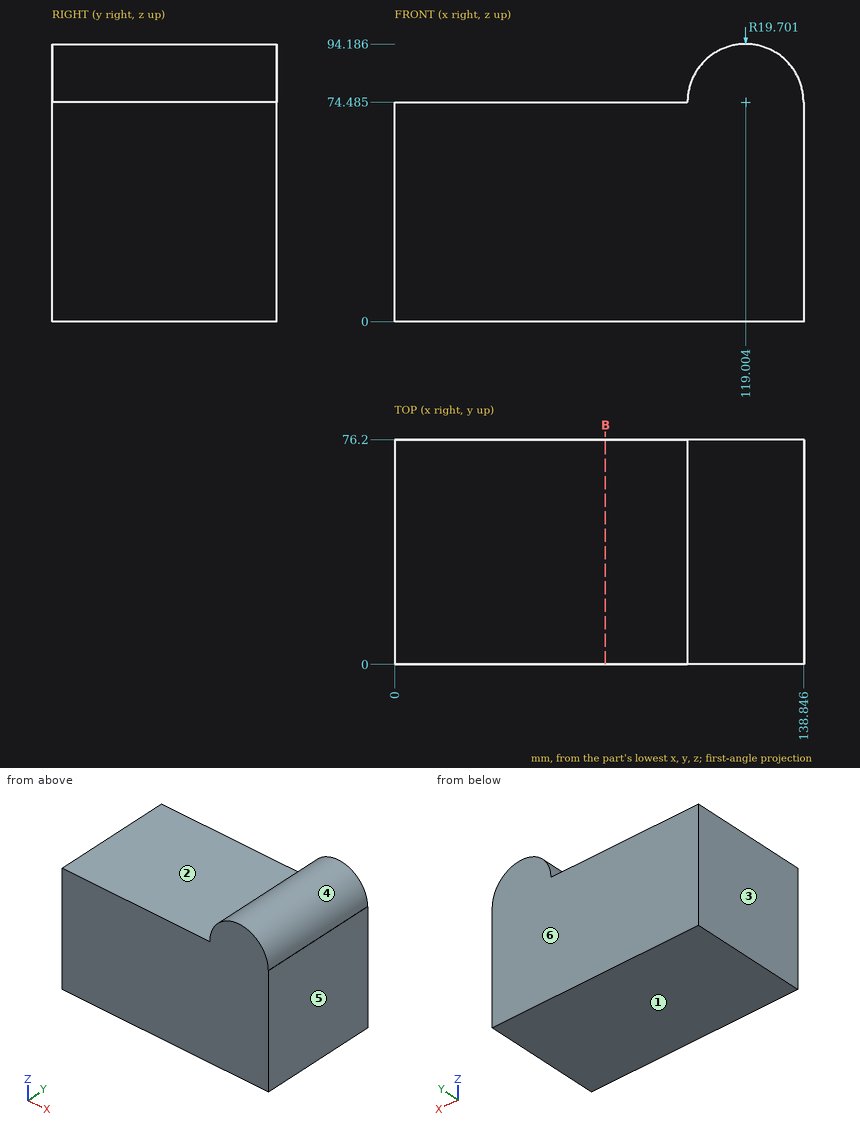
The drawing under review shows one solid part. Ordinate dimensions are in mm from its lowest x, y, z. A direction names the side the tool comes from. Round coordinates to 2 decimals unless told otherwise and drop trailing zeros. Order: outer loops, then holes, each group sorted by start corner. A loop starts at its lowest first (then second) coordinate and runs counter-clockwise, first axis right, second up. Notation, with made-up numbers: (-24.75, 84) -> (-0.75, 84) arc R28 cw to (-0.75, 114) -> close; hole circle Ø7 at (26.25, 81.5). An arc over 180 degrees is marked (long way). Return JSON: item names as keys, results as strings.
1. Take a section at B-B (x = 71.5). Write out the cut boundary in (y, z) (1 decimal).
Answer block:
{"outline": "(0, 0) -> (76.2, 0) -> (76.2, 74.5) -> (0, 74.5) -> close"}
2. The part is to be moulded in two halves that separate along X. For the marked faces 3, 4, 5 and 6, say which applies: +X half, -X half, draft (parallel to the pull), parting line (faces both ways), or undercut.
Answer block:
{"face 3": "-X half", "face 4": "parting line", "face 5": "+X half", "face 6": "draft"}
3. Insertion check: P1, Ø12, axis at x = 117.5, y = 50.5, coming from the +Z side; P2, Ø23, axis at x = 51, y = 38, coming from the +Z side (1 decimal); P3, Ø1, axis at x = 102, y = 34, coming from the +Z side (1 decimal). Each pin has a flat end and moves straight along its axis. Give the tip position at first contact, or say it passes through.
Answer block:
{"P1": "stops at z = 94.19", "P2": "stops at z = 74.5", "P3": "stops at z = 85.2"}
4. For L1, parallel to Z at x = 78, y = 73.5 (1 decimal); L2, parallel to Z at x = 107.5, y = 56; L3, parallel to X at y = 66.5, z = 79.5 (1 decimal), list the stretches that pass through material, from the lowest coordinate up. Write a range as [from, to].
Answer block:
{"L1": "z = [0, 74.5]", "L2": "z = [0, 90.48]", "L3": "x = [100, 138.1]"}
5. For the marked faces 1 and 2, list the 3-axis set-ups (+Z, -Z, +X, -X, +Y, -Y) from which the entire face can be reached by the end or side of a thin tool; tool diameter is ignored.
Answer block:
{"face 1": "-Z, +X, -X, +Y, -Y", "face 2": "+Z, -X, +Y, -Y"}
